```python
from build123d import *

# Parameters (mm, degrees)
F0_W     = 106.930423
F0_H     = 77.881411
F0_W_2   = 89.901697
F0_H_2   = 62.355211
F1_DEPTH = 25.4
F2_W     = 106.974344
F2_H     = 77.493225
F3_DEPTH = 7.62


with BuildPart() as f1:
    # F0 (on Front) → F1 (new body)
    with BuildSketch(Plane.XZ):
        with Locations((0.751262, 1.126902)):
            Rectangle(F0_W, F0_H)
        with Locations((0.500841, 0.626057)):
            Rectangle(F0_W_2, F0_H_2, mode=Mode.SUBTRACT)
    extrude(amount=F1_DEPTH)

    # F2 (on Front) → F3 (join)
    with BuildSketch(Plane.XZ):
        with Locations((1.196621, 1.206798)):
            Rectangle(F2_W, F2_H)
    extrude(amount=-F3_DEPTH)


solid = f1.part
```
Design review of the part built by this model. Coordinates are the model's own, in mm. A direction names the side the tool comes from. Give positions to 0.01 mm unless a question says otherwise; leave off trailing zeros. Order: outer loops, then holes, each group sorted by start corner. A loop starts at its lowest first (then second) coordinate and runs counter-clockwise, first axis right, second up. Notation, with made-up numbers: (-37.5, -4.75) - (0.5, -4.75) arc R11 cw to (0.5, 1.25) - close; hole circle Ø1 at (43, 82.25). An arc over 180 degrees is marked (long way). Use a Markdown table: item, result. Add a question column.
(1) Add section B-B on x = -39.5. Give the boundary of the cut face in (y, z).
(2) Mouldability with a two-part tool opening along X and no side actions: class faces 5 (the face through (-52.291, 4, 1)), 6 (the face through (0, -13, -37.814)), 7 (the face through (45.452, -13, 0)) as +X half, -X half, draft (parallel to the pull), parting line (faces both ways), or undercut.
(3) Machinability: for faces 1 (the face through (0, -13, 31.804)), 2 (the face through (54.216, -13, 1)), 3 (the face through (0, 4, 39.953)), 4 (the face through (0, 4, -37.54)), which of the approach directions +Z, -Z, +X, -X, +Y, -Y give a long, thin tool a straight path to every point of the face, cutting with its end or side? Answer none if there is none.
(4) Add section C-C on z = -4. Give the boundary of the cut face in (x, y).
(5) Wall thickness on probe 1 along X at (y, z) = (-21.5, 11); probe 2 along Z at (x, y) = (-28, -14.5); probe 3 along Y at (x, z) = (37.5, -19): over which ranges is each line inside the solid? List them lowest first. Write a range as [from, to].
(6) Clearance check with flat-ended pins moving along their axes: P1, Ø4, axis at x = 22.5, z = -13.5, coming from the -Y side; P2, Ø7.5, axis at y = -14, z = 14, coming from the +X side; P3, Ø2.5, axis at x = 27.5, y = 3.5, coming from the -Z side. State where each tip first meets the part, or that it passes through.
(7) Add section A-A on y = -20. Give the boundary of the cut face in (x, z), then the cut area to 3 significant figures.
Report:
| question | item | result |
|---|---|---|
| 1 | outline | (-25.4, -37.81) - (0, -37.81) - (0, -37.54) - (7.62, -37.54) - (7.62, 39.95) - (0, 39.95) - (0, 40.07) - (-25.4, 40.07) - (-25.4, 31.8) - (0, 31.8) - (0, -30.55) - (-25.4, -30.55) - close |
| 2 | face 5 | -X half |
| 2 | face 6 | draft |
| 2 | face 7 | undercut |
| 3 | face 1 | -Y |
| 3 | face 2 | +Z, -Z, +X, -Y |
| 3 | face 3 | +Z, +X, -X, +Y |
| 3 | face 4 | -Z, +X, -X, +Y |
| 4 | outline | (-52.71, -25.4) - (-44.45, -25.4) - (-44.45, 0) - (45.45, 0) - (45.45, -25.4) - (54.22, -25.4) - (54.22, 0) - (54.68, 0) - (54.68, 7.62) - (-52.29, 7.62) - (-52.29, 0) - (-52.71, 0) - close |
| 5 | probe 1 | x = [-52.71, -44.45], [45.45, 54.22] |
| 5 | probe 2 | z = [-37.81, -30.55], [31.8, 40.07] |
| 5 | probe 3 | y = [0, 7.62] |
| 6 | P1 | stops at y = 0 |
| 6 | P2 | stops at x = 54.22 |
| 6 | P3 | stops at z = -37.54 |
| 7 | outline | (-52.71, -37.81) - (54.22, -37.81) - (54.22, 40.07) - (-52.71, 40.07) - close; hole (-44.45, -30.55) - (45.45, -30.55) - (45.45, 31.8) - (-44.45, 31.8) - close |
| 7 | area | 2,720 mm² |
